from build123d import *

# Parameters (mm, degrees)
SKETCH_1_W          = 7.8
SKETCH_1_H          = 5.08
EXTRUDE_1_DEPTH     = 7.8
SKETCH_2_R          = 1.9
CUT_EXTRUDE_1_DEPTH = 4.2
SKETCH_3_W          = 2.509058382
SKETCH_3_H          = 0.614954654
CUT_EXTRUDE_2_DEPTH = 0.5
SKETCH_4_R          = 1.25
EXTRUDE_1_2_DEPTH   = 3
SKETCH_5_W          = 0.5
SKETCH_5_H          = 4.98
SKETCH_5_W_2        = 1.5
CUT_EXTRUDE_3_DEPTH = 12.760170067


with BuildPart() as part:
    # 草图1 → Extrude 1 (new body)
    with BuildSketch(Plane(origin=(0, 0, 0), x_dir=(1, 0, 0), z_dir=(0, 1, 0))):
        Rectangle(SKETCH_1_W, SKETCH_1_H)
    extrude(amount=EXTRUDE_1_DEPTH)

    # 草图2 → 切除-拉伸1 (cut)
    with BuildSketch(Plane(origin=(0, 7.8, 0), x_dir=(1, 0, 0), z_dir=(0, 1, 0))):
        with Locations(Location((0, 0, 0), (0, 0, 270))):
            Circle(SKETCH_2_R)
    extrude(amount=-CUT_EXTRUDE_1_DEPTH, mode=Mode.SUBTRACT)

    # 草图3 → 切除-拉伸2 (cut)
    with BuildSketch(Plane(origin=(0, 3.6, 0), x_dir=(1, 0, 0), z_dir=(0, 1, 0))):
        Rectangle(SKETCH_3_W, SKETCH_3_H)
    extrude(amount=-CUT_EXTRUDE_2_DEPTH, mode=Mode.SUBTRACT)

    # 草图4 → Extrude 1 2 (add)
    with BuildSketch(Plane.XZ):
        with Locations(Location((0, 0, 0), (0, 0, 90))):
            Circle(SKETCH_4_R)
    extrude(amount=EXTRUDE_1_2_DEPTH)

    # 草图5 → 切除-拉伸3 (cut, through all)
    with BuildSketch(Plane(origin=(0, 7.8, 0), x_dir=(1, 0, 0), z_dir=(0, 1, 0))):
        with Locations((-3.65, -0.05)):
            Rectangle(SKETCH_5_W, SKETCH_5_H)
        with Locations((3.15, -0.05)):
            Rectangle(SKETCH_5_W_2, SKETCH_5_H)
    extrude(amount=-CUT_EXTRUDE_3_DEPTH, mode=Mode.SUBTRACT)


solid = part.part
Design review of the part built by this model. Coordinates are the model's own, in mm. A direction names the side the tool comes from. Give positions to 0.01 mm unless a question says otherwise; leave off trailing zeros. Write each loop counter-clockwise with the first axis right and the second up, starting at its lowest first coordinate (ties: lowest second). Pieces come first, ordered by that corner, then holes. Notation, with made-up numbers: M -34.5,86 L 22.5,86 A24 cw 22.5,104 Z; hole C 83.5,-36.5 d8. An arc over 180 degrees is marked long. Answer as a JSON object with one key per item and string values. Group by question number.
1) Mouldability with a two-part tool opening along Z and no side actions: class faces 1 (the face through (-0.728, 5.729, 1.755)), 2 (the face through (-1, 4, 2.54)), 3 (the face through (2.4, 4, 0)) as released by +Z, released by -Z, zero draft, split by the parting line, or undercut.
2) Tool access review of faces 4 (the face through (0, 4, -2.54)), 5 (the face through (-1, 0, -1)), 6 (the face through (-3.4, 4, 0)): name each direction out of +Z, -Z, +X, -X, +Y, -Y from which nothing blocks a thin tool from reaching the whole face with its end or side.
3) We need section D-D (y = -0.25). Give the boundary of the cut face in (x, z), and give its area (3 significant figures).
4) We need section A-A (y = 6.5). Give the boundary of the cut face in (x, z).
5) We need section B-B (z = 0). Give the boundary of the cut face in (x, y), and give its area (3 significant figures).
6) Clearance check with flat-ended pins moving along their axes: pin 1 Ø0.5 at (x, y) = (3, 4.5) entering from +Z; pin 2 Ø2.5 at (x, z) = (1.5, 1.5) entering from -Y; pin 3 Ø1 at (y, z) = (2, 2) entering from -X. State where each tip first meets the part, or that it passes through.
7) We need section C-C (x = 0). Give the boundary of the cut face in (y, z).
8) For line 1 along Z through (x, y) = (0, 3.5); line 2 along X through (y, z) = (5.2, 0); line 3 along X through (y, z) = (3.5, -1.6), list the stretches that pass through material, from the lowest coordinate up.
Answer key:
{
 "1": {"face 1": "undercut", "face 2": "released by +Z", "face 3": "zero draft"},
 "2": {"face 4": "-Z, +X, -X, +Y, -Y", "face 5": "-Y", "face 6": "+Z, -X, +Y, -Y"},
 "3": {"outline": "C 0,0 d2.5", "area": "4.91 mm²"},
 "4": {"outline": "M -3.9,-2.54 L 3.9,-2.54 L 3.9,-2.44 L 2.4,-2.44 L 2.4,2.54 L -3.4,2.54 L -3.4,-2.44 L -3.9,-2.44 Z; hole C 0,0 d3.8"},
 "5": {"outline": "M -3.4,0 L -1.25,0 L -1.25,-3 L 1.25,-3 L 1.25,0 L 2.4,0 L 2.4,7.8 L 1.9,7.8 L 1.9,3.6 L 1.25,3.6 L 1.25,3.1 L -1.25,3.1 L -1.25,3.6 L -1.9,3.6 L -1.9,7.8 L -3.4,7.8 Z", "area": "35.5 mm²"},
 "6": {"pin 1": "stops at z = -2.44", "pin 2": "stops at y = -3", "pin 3": "stops at x = -3.4"},
 "7": {"outline": "M -3,-1.25 L 0,-1.25 L 0,-2.54 L 7.8,-2.54 L 7.8,-1.9 L 3.6,-1.9 L 3.6,-0.31 L 3.1,-0.31 L 3.1,0.31 L 3.6,0.31 L 3.6,1.9 L 7.8,1.9 L 7.8,2.54 L 0,2.54 L 0,1.25 L -3,1.25 Z"},
 "8": {"line 1": "z = -2.54 to -0.31, 0.31 to 2.54", "line 2": "x = -3.4 to -1.9, 1.9 to 2.4", "line 3": "x = -3.4 to 2.4"}
}
